Geometry: final body of the model. Coordinates: model frame, mm. A direction names the side the tool comes from. Round coordinates to 2 decimals unless told otherwise and drop trailing zeros. Write each loop counter-clockwise with the first axis right and the second up, starting at its lowest first coordinate (ties: lowest second). Pieces come first, ordered by that corner, then holes. Notation, with made-up numbers: (20, 58) -> (75, 58) arc R29 ccw to (75, 93) -> close; hole circle Ø7 at (23.5, 73.25). An arc over 180 degrees is marked (long way). Use one line per item in the form item = value. Start each with the question number.
1. Cut plane C-C, the plane z = 0.75. Return the cut outline in (x, y).
2. Cut plane D-D, the plane z = -0.75. Return the cut outline in (x, y), plus the area to 3 significant figures.
3. Cut plane B-B, the plane x = 0.35. Return the cut outline in (y, z).
4. Cut plane A-A, the plane y = 0. Return the cut outline in (x, z).
5. Reachability of faces 1 (the face through (0, 0, -3)), 2 (the face through (-0.7, 0, 5)), 3 (the face through (0.7, 0, -1.5)) from +Z, -Z, +X, -X, +Y, -Y: full face, straight path, thin tool, end or side. Return the list, or none.
6. Line query: L1, parallel to Y at x = 0, z = -1.25; L2, parallel to Y at x = -0.45, z = 4.5; L3, parallel to X at y = 0.15, z = 5.5. Output: solid intervals per line, ascending.
Autodesk Inventor part; units mm, degrees
ref_plane "YZ Plane" through (0, 0, 0) normal (1, 0, 0) x (0, 1, 0)
ref_plane "XZ Plane" through (0, 0, 0) normal (0, 1, 0) x (-1, 0, 0)
ref_plane "XY Plane" through (0, 0, 0) normal (0, 0, 1) x (1, 0, 0)
sketch "Sketch1" plane through (0, 0, 0) normal (0, 0, 1) x (1, 0, 0)
  circle A0 centre (0, 0) radius 0.75
  dimension "d0" = 1.5
extrude "Extrusion1" add sketch "Sketch1" along normal blind 3.5
sketch "Sketch2" plane through (0, 0, 3.5) normal (0, 0, 1) x (1, 0, 0)
  circle A0 centre (0, 0) radius 0.75
  circle A1 centre (0, 0) radius 0.7
  dimension "d3" = 1.4
extrude "Extrusion2" add sketch "Sketch2" along normal blind 3 contours A1
sketch "Sketch3" plane through (0, 0, 0) normal (0, 0, -1) x (-1, 0, 0)
  circle A0 centre (0, 0) radius 0.75
  circle A1 centre (0, 0) radius 0.7
  dimension "d6" = 1.4
extrude "Extrusion3" add sketch "Sketch3" along normal blind 3 contours A1
thread "Thread1"
thread "Thread2"
properties part number "25 - Disc Arm 2" material "Bronze, Soft Tin"
Outcome:
q1.outline = circle Ø1.5 at (0, 0)
q2.outline = circle Ø1.4 at (0, 0)
q2.area = 1.54 mm^2
q3.outline = (-0.66, 0) -> (-0.61, 0) -> (-0.61, -3) -> (0.61, -3) -> (0.61, 0) -> (0.66, 0) -> (0.66, 3.5) -> (0.61, 3.5) -> (0.61, 6.5) -> (-0.61, 6.5) -> (-0.61, 3.5) -> (-0.66, 3.5) -> close
q4.outline = (-0.75, 0) -> (-0.7, 0) -> (-0.7, -3) -> (0.7, -3) -> (0.7, 0) -> (0.75, 0) -> (0.75, 3.5) -> (0.7, 3.5) -> (0.7, 6.5) -> (-0.7, 6.5) -> (-0.7, 3.5) -> (-0.75, 3.5) -> close
q5.face_1 = -Z, +X, -X, +Y, -Y
q5.face_2 = +Z
q5.face_3 = -Z
q6.L1 = -0.7 to 0.7
q6.L2 = -0.54 to 0.54
q6.L3 = -0.68 to 0.68
